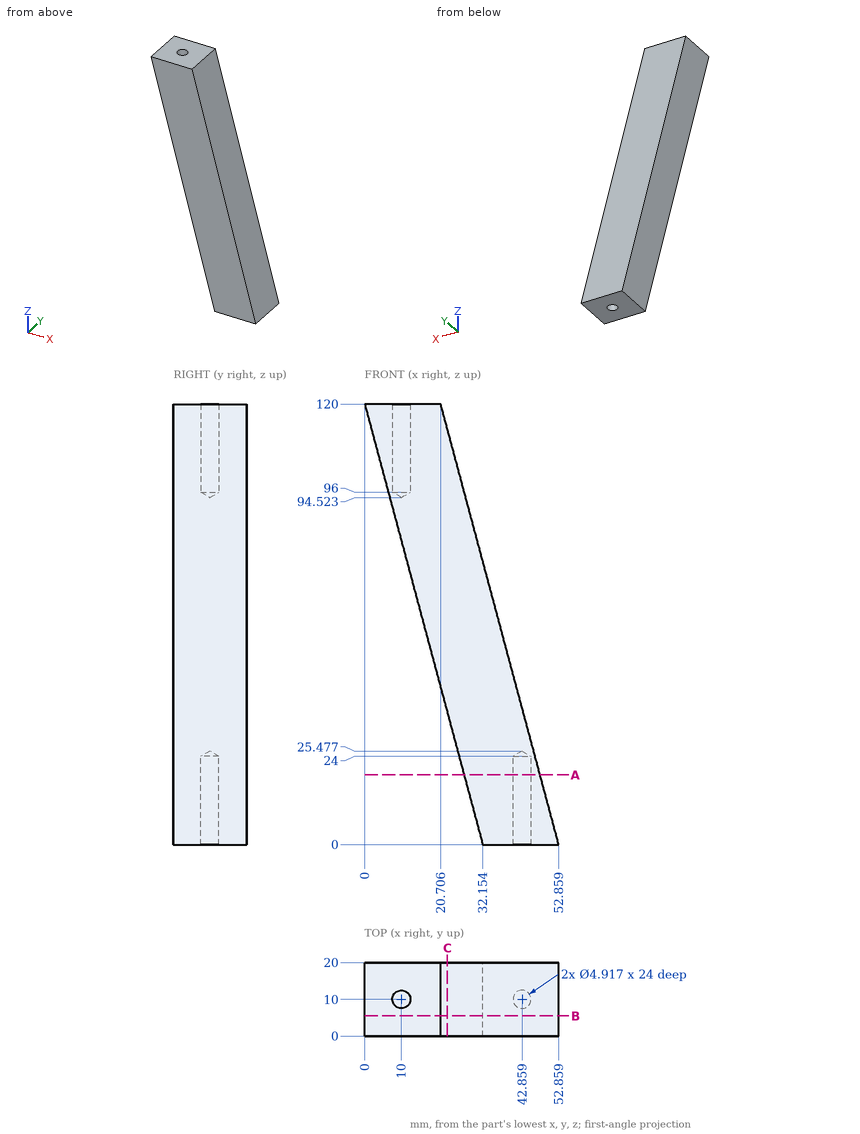
Answer from the drawing. Dimensions are ordinates in mm from the lowest x, y and z of the part. Give positions to 0.01 mm unless a question says otherwise; leave off trailing zeros. Order: outer loops, then holes, each group sorted by start corner. A loop starts at its lowest first (then second) coordinate and runs counter-clockwise, first axis right, second up. Notation, with made-up numbers: (-2.5, 12) -> (55.5, 12) arc R16 cw to (55.5, 21) -> close; hole circle Ø7 at (29.5, 32). An arc over 180 degrees is marked (long way). One line per item, written item: value. Start each with the question number.
(1) The part is cut by section C-C (x = 22.5). Determine the outline of the cut face in (y, z), and give its area (3 significant figures).
(2) The part is cut by section A-A (z = 19). Determine the outline of the cut face in (x, y).
(3) The part is cut by section B-B (y = 5.5). Determine the outline of the cut face in (x, z) (1 decimal).
(4) Straight lines are drawn through the part: L1, parallel to Y at x = 10, z = 112.75; L2, parallel to X at y = 10, z = 106.5; L3, parallel to X at y = 10, z = 10.25. For each, find the intervals that lie inside material, in ascending order.
(5) Flat-ended cylindrical pins translate along their axes: P1, Ø3, axis at x = 42.86, y = 10, coming from the -Z side (1 decimal); P2, Ø12, axis at y = 16.5, z = 53.5, coming from the -X side; P3, Ø12, axis at y = 5.5, z = 30, coming from the +X side. Find the tip coordinate at first contact, or state that the pin passes through.
Taken from the geometry:
1. outline: (0, 36.03) -> (20, 36.03) -> (20, 113.3) -> (0, 113.3) -> close
1. area: 1,550 mm^2
2. outline: (27.06, 0) -> (47.77, 0) -> (47.77, 20) -> (27.06, 20) -> close; hole circle Ø4.92 at (42.86, 10)
3. outline: (0, 120) -> (32.2, 0) -> (52.9, 0) -> (20.7, 120) -> close
4. L1: 0 to 7.54, 12.46 to 20
4. L2: 3.62 to 7.54, 12.46 to 24.32
4. L3: 29.41 to 40.4, 45.32 to 50.11
5. P1: z = 24.6
5. P2: x = 16.21
5. P3: x = 46.43
